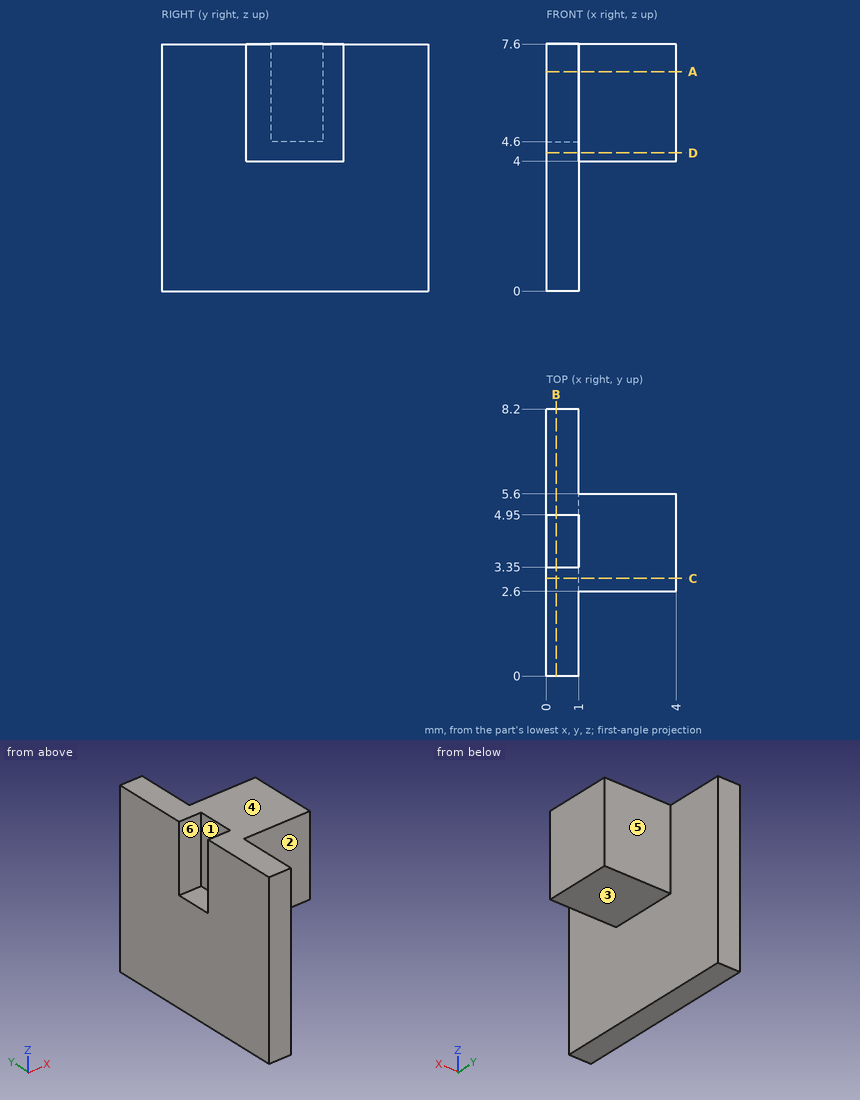
Answer from the drawing. Dimensions are ordinates in mm from the lowest x, y and z of the part. A direction names the side the tool comes from. Give positions to 0.01 mm unless a question says otherwise; leave off trailing zeros. Loops run counter-clockwise (first coordinate to the right, second up) from the corner with the lowest first, then second, coordinate; pieces in that order, holes last. Notation, with made-up numbers: M 1,63 L 28,63 A32 cw 28,102 Z; hole C 23.5,69.25 d1. An arc over 180 degrees is marked long. One line per item, written item: value.
Q1. Find the intervals of material crossed by line 1 (Y direction, x = 0.4, z = 6.75); line 2 (Z direction, x = 1.6, y = 4.5); line 3 (Y direction, x = 2.65, z = 6.75), in increasing order. Write a range as from..to.
Working result:
line 1: y = 0..3.35, 4.95..8.2
line 2: z = 4..7.6
line 3: y = 2.6..5.6
Q2. A cutting plane is placed at C-C on y = 3. Determine the outline of the cut face in (x, z).
Working result:
outline: M 0,0 L 1,0 L 1,4 L 4,4 L 4,7.6 L 0,7.6 Z
Q3. A cutting plane is placed at A-A on z = 6.75. Determine the outline of the cut face in (x, y).
Working result:
outline: M 0,0 L 1,0 L 1,2.6 L 4,2.6 L 4,5.6 L 1,5.6 L 1,8.2 L 0,8.2 L 0,4.95 L 1,4.95 L 1,3.35 L 0,3.35 Z
Q4. A cutting plane is placed at D-D on z = 4.25. Determine the outline of the cut face in (x, y), then the cut area to 3 significant figures.
Working result:
outline: M 0,0 L 1,0 L 1,2.6 L 4,2.6 L 4,5.6 L 1,5.6 L 1,8.2 L 0,8.2 Z
area: 17.2 mm^2
Q5. A cutting plane is placed at B-B on x = 0.3. Determine the outline of the cut face in (y, z), then the cut area to 3 significant figures.
Working result:
outline: M 0,0 L 8.2,0 L 8.2,7.6 L 4.95,7.6 L 4.95,4.6 L 3.35,4.6 L 3.35,7.6 L 0,7.6 Z
area: 57.5 mm^2
Q6. For the marked faces 1, 2 and 3, determine the directions among +Z, -Z, +X, -X, +Y, -Y from which every point of the face is accessible in a straight line to the end or side of a thin tool.
Working result:
face 1: +Z, -X
face 2: +Z, -Z, +X, -Y
face 3: -Z, +X, +Y, -Y
Q7. Flat-ended cylindrical pins translate along their axes: P1, Ø1, axis at x = 2.5, z = 4, coming from the +Y side; P2, Ø0.5, axis at x = 0.5, y = 4, coming from the +Z side. Find the tip coordinate at first contact, or state that the pin passes through.
Working result:
P1: stops at y = 5.6
P2: stops at z = 4.6
Q8. Determine the mould class of the marked faces 4, 5 and 6 for opening direction Y: +Y half, -Y half, draft (parallel to the pull), parting line (faces both ways), or undercut.
Working result:
face 4: draft
face 5: +Y half
face 6: undercut
